```python
from build123d import *

# Parameters (mm, degrees)
F0_R     = 6
F1_DEPTH = 200
F2_R     = 6
F0_W     = 25
F0_H     = 25
F3_DEPTH = 9


with BuildPart() as f1:
    # F0 (on Front) → F1 (new body)
    with BuildSketch(Plane.XZ):
        Circle(F0_R)
    extrude(amount=-F1_DEPTH)

    # F2 (on face) + F0 (on Front) → F3 (join)
    with BuildSketch(Plane.XZ):
        Circle(F2_R)
    with BuildSketch(Plane.XZ):
        Rectangle(F0_W, F0_H)
        Circle(F0_R, mode=Mode.SUBTRACT)
    extrude(amount=F3_DEPTH)


solid = f1.part
```
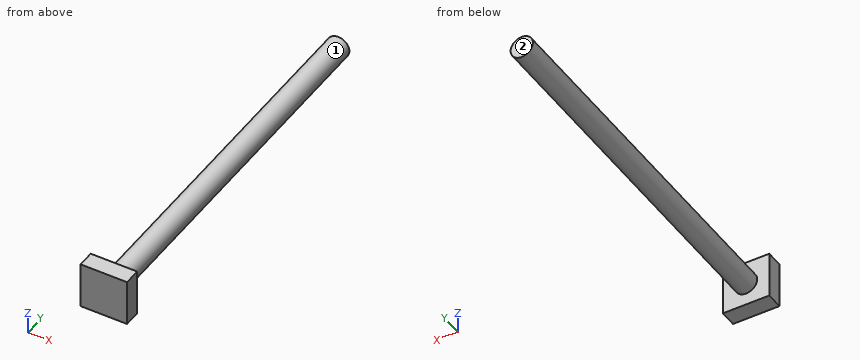
Geometry check sheet. Reference: the model listing, model coordinates, mm. Face numbers are marked on the shaded views. A direction names the side the tool comes from. Give positions to 0.01 mm unless a question says otherwise; leave off trailing zeros. Write each loop counter-clockwise with the first axis right and the second up, starting at its lowest first coordinate (ties: lowest second). Pieces come first, ordered by that corner, then holes. Notation, with made-up numbers: (-23, 7.5) -> (0, 7.5) arc R17 cw to (0, 19.5) -> close; hole circle Ø7 at (10.25, 7.5). An arc over 180 degrees is marked (long way). Use one line per item in the form item = value.
Item 1: Sectioned sample at B-B on z = 0. Enter the section's corners in (x, y).
Results list:
outline = (-12.5, -9) -> (12.5, -9) -> (12.5, 0) -> (6, 0) -> (6, 200) -> (-6, 200) -> (-6, 0) -> (-12.5, 0) -> close
Item 2: Sectioned sample at C-C on y = 128.5. Enter the section's corners in (x, z), plus the area to 3 significant figures.
Results list:
outline = circle Ø12 at (0, 0)
area = 113 mm2
Item 3: Sectioned sample at A-A on x = 0. Enter the section's corners in (y, z), plus the area to 4 significant figures.
Results list:
outline = (-9, -12.5) -> (0, -12.5) -> (0, -6) -> (200, -6) -> (200, 6) -> (0, 6) -> (0, 12.5) -> (-9, 12.5) -> close
area = 2,625 mm2
Item 4: Scan lines: line 1 (Y direction, x = -10.75, z = 8.5); line 2 (X direction, y = 142.5, z = 0.5); line 3 (X direction, y = 142, z = 5.5). Record each from-to range of solid material in increasing order.
Results list:
line_1 = -9 to 0
line_2 = -5.98 to 5.98
line_3 = -2.4 to 2.4
Item 5: Depth check by flat-ended pin: pin 1 Ø3 at (x, y) = (4, 57) entering from +Z; pin 2 Ø1.5 at (y, z) = (50.5, 2) entering from +X; pin 3 Ø5 at (x, y) = (-3, 100.5) entering from -Z. Enter the tip coordinate at first touch or a pass-through.
Results list:
pin_1 = 5.45
pin_2 = 5.87
pin_3 = -5.98
Item 6: Access from +Z, -Z, +X, -X, +Y, -Y to the whole of each face (thin tool, end or side, straight path). Record for the marked faces 1 and 2.
Results list:
face_1 = +Y
face_2 = +Z, -Z, +X, -X, +Y
Item 7: Sectioned sample at D-D on x = -9. Enter the section's corners in (y, z), plus the area to 3 significant figures.
Results list:
outline = (-9, -12.5) -> (0, -12.5) -> (0, 12.5) -> (-9, 12.5) -> close
area = 225 mm2
